Autodesk Inventor part; units mm, degrees
ref_plane "YZ Plane" through (0, 0, 0) normal (1, 0, 0) x (0, 1, 0)
ref_plane "XZ Plane" through (0, 0, 0) normal (0, 1, 0) x (-1, 0, 0)
ref_plane "XY Plane" through (0, 0, 0) normal (0, 0, 1) x (1, 0, 0)
sketch "Szkic1" plane through (0, 0, 0) normal (0, 0, 1) x (1, 0, 0)
  line L0 (-10.1243, 0) -> (60.0207, 0)
  line L1 (0, -10.1243) -> (0, 60.0207)
  line L2 (0, 50) -> (0, 0.5)
  line L3 (0.5, 0) -> (50, 0)
  line L4 (50, 2) -> (2.5, 2)
  line L5 (2, 2.5) -> (2, 50)
  line L6 (2, 50) -> (0, 50)
  line L7 (50, 0) -> (50, 2)
  arc A0 (2, 2.5) -> (2.5, 2) centre (2.5, 2.5) ccw
  arc A1 (0, 0.5) -> (0.5, 0) centre (0.5, 0.5) ccw
  point P0 (0, 0)
  dimension "d0" = 2
  dimension "d2" = 2
  dimension "d3" = 50
  dimension "d4" = 50
  dimension "d5" = 0.5
extrude "Wyciągnięcie proste1" add sketch "Szkic1" along normal blind 300 contours A1 L1 L6 L5 A0 L4 L7 L0
properties part number "kątownik 1" material "Aluminium 6061"
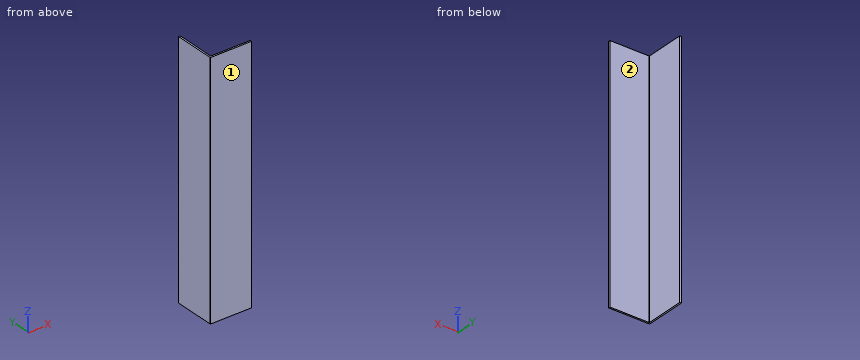
The model under review builds one solid part; all positions refer to its coordinate system, in mm. Face numbers are marked on the shaded views. A direction names the side the tool comes from. Give positions to 0.01 mm unless a question says otherwise; leave off trailing zeros. Loops run counter-clockwise (first coordinate to the right, second up) from the corner with the lowest first, then second, coordinate; pieces in that order, holes last. Notation, with made-up numbers: (-35, 4.5) - (-9, 4.5) arc R23 ccw to (-9, 14.5) - close; hole circle Ø2 at (3.5, -6.75). An arc over 180 degrees is marked (long way). Answer as a JSON object with one key per item and string values.
Q1. Insertion check: pin 1 (6 mm diameter, centred on x = 7, z = 217, fed in from +Y); pin 2 (24 mm diameter, centred on y = 31.5, z = 121.5, fed in from +X). Each pin has a flat end and moves straight along its axis. Give the tip position at first contact, or say it passes through.
Worked out:
{"pin 1": "stops at y = 2", "pin 2": "stops at x = 2"}
Q2. Add section B-B on y = 37. State the section outline as (x, z) points.
Worked out:
{"outline": "(0, 0) - (2, 0) - (2, 300) - (0, 300) - close"}
Q3. Add section A-A on z = 229. State the section outline as (x, y) points.
Worked out:
{"outline": "(0, 0.5) arc R0.5 ccw to (0.5, 0) - (50, 0) - (50, 2) - (2.5, 2) arc R0.5 cw to (2, 2.5) - (2, 50) - (0, 50) - close"}
Q4. For the marked faces 1 and 2, list the 3-axis set-ups (+Z, -Z, +X, -X, +Y, -Y) from which the entire face can be reached by the end or side of a thin tool; tool diameter is ignored.
Worked out:
{"face 1": "+Z, -Z, +X, -X, -Y", "face 2": "+Z, -Z, +X, +Y"}
Q5. To check wall thickness, follow line 1 along X through (y, z) = (17.5, 277). State the ranges of the line that lie inside material, in increasing order.
Worked out:
{"line 1": "x = 0 to 2"}
